```python
from build123d import *

# Parameters (mm, degrees)
ESQUISSE1_R                  = 0.7
BOSS_EXTRU_1_DEPTH           = 1.3
BOSS_EXTRU_2_DEPTH           = 0.1
CHANFREIN1_SIZE              = 0.1
CONG_1_R                     = 0.3
ESQUISSE3_R                  = 0.35
BOSS_EXTRU_3_DEPTH           = 0.7
CHANFREIN2_SIZE              = 0.25
CONG_2_R                     = 0.1
CONG_3_R                     = 0.1
ENL_V_MAT_EXTRU_1_DEPTH      = 0.7
ENL_V_MAT_EXTRU_1_DEPTH_BACK = 0.7
ESQUISSE4_R                  = 0.05
CONG_4_R                     = 0.1
ESQUISSE5_R                  = 0.225
ENL_V_MAT_EXTRU_2_DEPTH      = 0.5
CONG_5_R                     = 0.2
ECHELLE1_SCALE               = 10


with BuildPart() as part:
    # Esquisse1 → Boss.-Extru.1 (new body)
    with BuildSketch(Plane(origin=(0, 0, 0), x_dir=(1, 0, 0), z_dir=(0, 1, 0))):
        Polygon((0.501147742, 0.810154887), (-0.451040842, 0.839084119), (-0.952188584, 0.028929232), (-0.501147742, -0.810154887), (0.451040842, -0.839084119), (0.952188584, -0.028929232), align=None)
        with Locations(Location((0, 0, 0), (0, 0, 270))):
            Circle(ESQUISSE1_R, mode=Mode.SUBTRACT)
    extrude(amount=BOSS_EXTRU_1_DEPTH)

    # Esquisse2 → Boss.-Extru.2 (add)
    with BuildSketch(Plane.XZ):
        Polygon((0.501147742, -0.810154887), (0.952188584, 0.028929232), (0.451040842, 0.839084119), (-0.501147742, 0.810154887), (-0.952188584, -0.028929232), (-0.451040842, -0.839084119), align=None)
    extrude(amount=BOSS_EXTRU_2_DEPTH)

    # Chanfrein1
    chanfrein1_edges = [part.edges().sort_by_distance(p)[0] for p in [
        (-0.701614713, 1.3, -0.434006676),
        (-0.726668163, 1.3, 0.390612827),
        (-0.02505345, 1.3, 0.824619503),
        (0.701614713, 1.3, 0.434006676),
        (0.02505345, -0.1, -0.824619503),
        (0.726668163, -0.1, -0.390612827),
        (0.701614713, -0.1, 0.434006676),
        (-0.02505345, -0.1, 0.824619503),
        (-0.726668163, -0.1, 0.390612827),
        (-0.701614713, -0.1, -0.434006676),
        (0.726668163, 1.3, -0.390612827),
        (0.02505345, 1.3, -0.824619503),
    ]]
    chamfer(chanfrein1_edges, length=CHANFREIN1_SIZE)

    # Congé1
    cong_1_edges = [part.edges().sort_by_distance(p)[0] for p in [
        (0.501147742, 0.6, -0.810154887),
        (-0.451040842, 0.6, -0.839084119),
        (0.952188584, 0.6, 0.028929232),
        (0.451040842, 0.6, 0.839084119),
        (-0.501147742, 0.6, 0.810154887),
        (-0.952188584, 0.6, -0.028929232),
    ]]
    fillet(cong_1_edges, radius=CONG_1_R)

    # Esquisse3 → Boss.-Extru.3 (add)
    with BuildSketch(Plane(origin=(0, -0.1, 0), x_dir=(-1, 0, 0), z_dir=(0, -1, 0))):
        with Locations(Location((0, 0, 0), (0, 0, 90))):
            Circle(ESQUISSE3_R)
    extrude(amount=BOSS_EXTRU_3_DEPTH)

    # Chanfrein2
    chanfrein2_edges = [part.edges().sort_by_distance(p)[0] for p in [
        (0, -0.8, 0.35),
    ]]
    chamfer(chanfrein2_edges, length=CHANFREIN2_SIZE)

    # Congé2
    # the kernel refuses this fillet: 0.1 mm, written as the material it takes off along each edge
    with BuildSketch(Plane(origin=(0, 1.3, 0), x_dir=(0, 0, 1), z_dir=(-1, 0, 0))) as cong_2_piece_1:
        with BuildLine():
            CenterArc((0.7 + CONG_2_R, -CONG_2_R), CONG_2_R, 90, 90)
            Line((0.7, -CONG_2_R), (0.7, 0))
            Line((0.7, 0), (0.7 + CONG_2_R, 0))
        make_face()
    revolve(axis=Axis((0, 1.3, 0), (0, 1, 0)), mode=Mode.SUBTRACT)

    # Congé3
    cong_3_edges = [part.edges().sort_by_distance(p)[0] for p in [
        (0, -0.1, 0.35),
    ]]
    fillet(cong_3_edges, radius=CONG_3_R)

    # Esquisse4 → Enlèv. mat.-Extru.1 (cut, two sides: drawn at the far end of the back side and taken through both)
    with BuildSketch(Plane(origin=(0, 0, 0), x_dir=(0, 0, -1), z_dir=(1, 0, 0)).offset(-ENL_V_MAT_EXTRU_1_DEPTH_BACK)):
        with Locations(Location((0, -0.68, 0), (0, 0, 297.173904779))):
            Circle(ESQUISSE4_R)
    extrude(amount=ENL_V_MAT_EXTRU_1_DEPTH + ENL_V_MAT_EXTRU_1_DEPTH_BACK, mode=Mode.SUBTRACT)

    # Congé4
    cong_4_edges = [part.edges().sort_by_distance(p)[0] for p in [
        (0, -0.55, 0.35),
    ]]
    fillet(cong_4_edges, radius=CONG_4_R)

    # Esquisse5 → Enlèv. mat.-Extru.2 (cut)
    with BuildSketch(Plane(origin=(0, 0, 0), x_dir=(1, 0, 0), z_dir=(0, 1, 0))):
        with Locations(Location((0, 0, 0), (0, 0, 270))):
            Circle(ESQUISSE5_R)
    extrude(amount=-ENL_V_MAT_EXTRU_2_DEPTH, mode=Mode.SUBTRACT)

    # Congé5
    cong_5_edges = [part.edges().sort_by_distance(p)[0] for p in [
        (0, 0, -0.225),
    ]]
    fillet(cong_5_edges, radius=CONG_5_R)


with BuildPart() as part_1:
    # Echelle1: scaled about (0, 0, 0)
    add(part.part.scale(ECHELLE1_SCALE))


solid = part_1.part
```
The listing builds one solid part. Answer for the finished solid, in the listing's coordinates (mm). A direction names the side the tool comes from. Give positions to 0.01 mm unless a question says otherwise; leave off trailing zeros. Order: outer loops, then holes, each group sorted by start corner. A loop starts at its lowest first (then second) coordinate and runs counter-clockwise, first axis right, second up. Notation, with made-up numbers: (30.25, -18) - (81.25, -18) arc R23 ccw to (81.25, -8) - close; hole circle Ø11 at (47, -24). An arc over 180 degrees is marked (long way). Use one line per item in the form item = value. Start each with the question number.
(1) A cutting plane is placed at B-B, the plane y = -6.8. Write down the section's boundary in (x, z).
(2) The mould has two halves that part along Z. Classify faces 3 (the cylindrical face through (-6.834, 5.916, -1.517)), 4 (the flat face through (6.85, 12.51, -3.61)), 5 (the flat face through (7.04, 6.08, 4.3)): released by +Z, released by -Z, zero draft, split by the parting line, or undercut.
(3) For faces 1 (the cylindrical face through (0.676, -3.479, 2.146)), 2 (the flat face through (7.25, 6.08, -3.94)), determine the directions among +Z, -Z, +X, -X, +Y, -Y from which every point of the face is accessible in a straight line to the end or side of a thin tool.
(4) Flat-ended cylindrical pins translate along their axes: pin 1 Ø3 at (x, y) = (0, 5.5) entering from +Z; pin 2 Ø2 at (x, z) = (-7, -3) entering from -Y; pin 3 Ø10 at (x, z) = (4, -4.5) entering from +Y; pin 4 Ø1.5 at (x, z) = (-3.5, 0) entering from -Y. Find the tip coordinate at first contact, or state that the pin passes through.
(5) Consider line 1 (X direction, y = 8.5, z = 0); line 2 (Y direction, x = -1.3, z = 0); line 3 (Y direction, x = -6.25, z = 2). Determine where each line is inside the solid, lowest interval first. Write a range as from..to.
(6) A cutting plane is placed at A-A, the plane y = 8.25. Write down the section's boundary in (x, z).
(7) A cutting plane is placed at C-C, the plane y = -2.75. Write down the section's boundary in (x, z).
Ans:
q1.outline = (-2.14, -0.5) arc R2.2 ccw to (2.14, -0.5) - close; (-2.14, 0.5) - (2.14, 0.5) arc R2.2 ccw to start
q2.face_3 = undercut
q2.face_4 = released by -Z
q2.face_5 = released by +Z
q3.face_1 = +Y
q3.face_2 = -Z, +X, +Y, -Y
q4.pin_1 = 8.3
q4.pin_2 = -1
q4.pin_3 = 13
q4.pin_4 = -6.25
q5.line_1 = -9.05..-7, 7..9.05
q5.line_2 = -7.7..-7.3, -6.3..-5
q5.line_3 = -1..0
q6.outline = (-8.7, 1.24) arc R3 ccw to (-8.61, -1.76) - (-5.42, -6.92) arc R3 ccw to (-2.78, -8.34) - (3.28, -8.15) arc R3 ccw to (5.83, -6.58) - (8.7, -1.24) arc R3 ccw to (8.61, 1.76) - (5.42, 6.92) arc R3 ccw to (2.78, 8.34) - (-3.28, 8.15) arc R3 ccw to (-5.83, 6.58) - close; hole circle Ø14 at (0, 0)
q7.outline = circle Ø7 at (0, 0); hole circle Ø4.5 at (0, 0)
